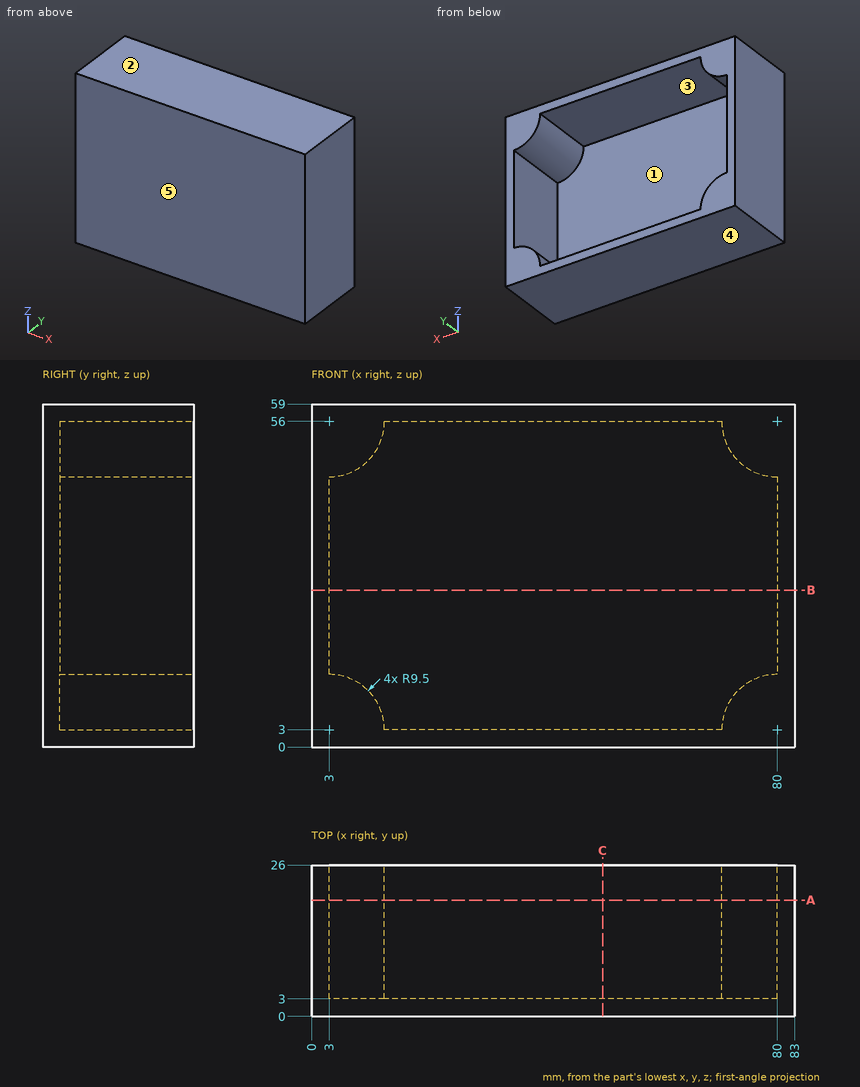
For this review, use the dimensioned drawing (mm, ordinates from the lowest corner) and the shaded views. A direction names the side the tool comes from. Coordinates: 2 decimals unless noted, no trailing zeros. Loops run counter-clockwise (first coordinate to the right, second up) from the corner with the lowest first, then second, coordinate; pieces in that order, holes last. Notation, with made-up numbers: (66, 8) -> (71, 8) arc R16 ccw to (71, 14) -> close; hole circle Ø4 at (-17, 56). An arc over 180 degrees is marked (long way). Return JSON: item names as keys, results as strings. Group by question number.
(1) To check wall thickness, follow L1, parallel to Z at x = 59, y = 20.25; L2, parallel to X at y = 22, z = 19; L3, parallel to Y at x = 23, z = 24. State the ranges of each line that lie inside material, in increasing order.
(2) Consider section A-A, the plane y = 20. Give the boundary of the cut face in (x, z), plus the area to 3 significant figures.
(3) For pin 1 Ø2 at (x, z) = (65.5, 48) entering from +Y, flat-tipped, find the tip position at first contact; note if it passes through.
(4) Tool access review of the marked faces 1 and 2: name each direction out of +Z, -Z, +X, -X, +Y, -Y from which nothing blocks a thin tool from reaching the whole face with its end or side.
(5) Mouldability with a two-part tool opening along Z and no side actions: class the marked faces 3, 4 and 5 as pulls with the +Z half, pulls with the -Z half, needs draft (parallel to the pull), parting line crosses it, or undercut.
(6) Consider section B-B, the plane z = 27. Give the boundary of the cut face in (x, y).
(7) Consider section C-C, the plane x = 50. Give the boundary of the cut face in (y, z).
Results below:
{
 "1": {"L1": "z = 0 to 3, 56 to 59", "L2": "x = 0 to 3, 80 to 83", "L3": "y = 0 to 3"},
 "2": {"outline": "(0, 0) -> (83, 0) -> (83, 59) -> (0, 59) -> close; hole (3, 12.5) arc R9.5 cw to (12.5, 3) -> (70.5, 3) arc R9.5 cw to (80, 12.5) -> (80, 46.5) arc R9.5 cw to (70.5, 56) -> (12.5, 56) arc R9.5 cw to (3, 46.5) -> close", "area": "1,100 mm2"},
 "3": {"pin 1": "stops at y = 3"},
 "4": {"face 1": "+Y", "face 2": "+Z, +X, -X, +Y, -Y"},
 "5": {"face 3": "undercut", "face 4": "pulls with the -Z half", "face 5": "needs draft"},
 "6": {"outline": "(0, 0) -> (83, 0) -> (83, 26) -> (80, 26) -> (80, 3) -> (3, 3) -> (3, 26) -> (0, 26) -> close"},
 "7": {"outline": "(0, 0) -> (26, 0) -> (26, 3) -> (3, 3) -> (3, 56) -> (26, 56) -> (26, 59) -> (0, 59) -> close"}
}
